from build123d import *

# Parameters (mm, degrees)
BOSS_EXTRUDE1_DEPTH = 88
SKETCH5_W           = 120.314234724
SKETCH5_H           = 205.924557391
CUT_EXTRUDE1_DEPTH  = 88
CUT_EXTRUDE2_REACH  = 78.774


with BuildPart() as part:
    # Sketch2 → Boss-Extrude1 (new body)
    with BuildSketch(Plane.XY):
        Polygon((21.738330866, 28.073521819), (21.738330866, -43.926478181), (-19.131432817, -43.926478181), (-19.989175059, -37.823325008), (7.738330866, -33.926478181), (0.362156515, 18.557729462), (-6.569719966, 17.583517755), (-8.043993893, 28.073521819), align=None)
    extrude(amount=-BOSS_EXTRUDE1_DEPTH)

    # Sketch5 → Cut-Extrude1 (cut)
    with BuildSketch(Plane(origin=(19.710307893, 24.555901932, -20.242027268), x_dir=(-0.850144649, 0.406300724, -0.33492357), z_dir=(-0.526549216, -0.655996394, 0.540753784))):
        with Locations((18.13624664, 41.178747918)):
            Rectangle(SKETCH5_W, SKETCH5_H)
    extrude(amount=-CUT_EXTRUDE1_DEPTH, mode=Mode.SUBTRACT)

    # Cut-Extrude2: up to this face of the body (flat: up to its plane)
    cut_extrude2_end = Plane(part.part.faces().sort_by_distance((4.446485826, -10.503783654, -37.636714234))[0])
    # Sketch6 → Cut-Extrude2 (cut, up to the picked face)
    with BuildSketch(Plane(origin=(19.710307893, 24.555901932, -20.242027268), x_dir=(0.850144649, -0.406300724, 0.33492357), z_dir=(0.526549216, 0.655996394, -0.540753784)), mode=Mode.PRIVATE) as cut_extrude2_sk1:
        with BuildLine():
            Line((-1.614496573, 26.946007892), (-1.614496573, 48.946007892))
            ThreePointArc((-1.614496573, 48.946007892), (-5.614496573, 52.946007892), (-9.614496573, 48.946007892))
            Line((-9.614496573, 48.946007892), (-9.614496573, 26.946007892))
            ThreePointArc((-9.614496573, 26.946007892), (-5.614496573, 22.946007892), (-1.614496573, 26.946007892))
        make_face()
    cut_extrude2_tool1 = split(extrude(cut_extrude2_sk1.sketch, amount=-CUT_EXTRUDE2_REACH, mode=Mode.PRIVATE), bisect_by=cut_extrude2_end, keep=Keep.BOTH, mode=Mode.PRIVATE)
    add(cut_extrude2_tool1.solids().sort_by_distance((14.937174, 2.700657, -51.4027))[0], mode=Mode.SUBTRACT)


solid = part.part
Here's how the part is built. I have some questions about the finished solid (model axes, mm). A direction names the side the tool comes from. Round coordinates to 2 decimals unless told otherwise and drop trailing zeros. Loops run counter-clockwise (first coordinate to the right, second up) from the corner with the lowest first, then second, coordinate; pieces in that order, holes last. Notation, with made-up numbers: M 52,40.5 L 75,40.5 A20 ccw 75,76.5 Z; hole C 37,31 d1. An arc over 180 degrees is marked long. Write each question's results on one line, items separated by ' | '. Start each with the question number.
(1) I want a section at A-A (z = -24). Please give me the cut outline in (x, y).
(2) Thinking about a two-plate mould opening in Z: for faces 1 (the flat face through (3, 28.074, -16)), 2 (the flat face through (10, -7, 0)), 3 (the cylindrical face through (10.644, 4.875, -34.03)), 4 (the flat face through (10.365, 2.582, -55.999)), which applies, pulls with the +Z half, pulls with the -Z half, needs draft (parallel to the pull), parting line crosses it, or undercut?
(3) I want a section at B-B (y = -30). Please give me the cut outline in (x, z).
(4) On a 3-axis mill with a long thin cutter (end or side, diameter ignored), from which of +Z, -Z, +X, -X, +Y, -Y can I reach the whole of each face in a straight line? I mean faces 5 (the flat face through (-3.055, 18.077, -26.765)), 6 (the flat face through (-7.297, 22.755, -26.765)), 7 (the flat face through (11.414, -7.452, -42.834)), 8 (the flat face through (21.738, -15, -34)). Say none if no direction works.
(5) I want a section at C-C (x = -14.5). Please give me the cut outline in (y, z), then the cut area to 3 significant figures.
(6) If I drill on probe 1 along Y at (x, z) = (8, -43.5); probe 2 along X at (y, z) = (1, -27); probe 3 along X at (y, z) = (1.5, -37.5), over which ranges is the centre line in solid material (lowest first)? Write a range as from..to.
(7) I want a section at D-D (z = -71). Please give me the cut outline in (x, y).
(8) Will these pins go through, and if not, where does the flat tip stop? P1, Ø10, axis at y = -26, z = -14, coming from the -X side; P2, Ø6, axis at x = -13, z = -42.5, coming from the +Y side; P3, Ø5, axis at y = -24.5, z = -25.5, coming from the -X side.
Solved:
1) outline: M -19.99,-37.82 L -19.13,-43.93 L 21.74,-43.93 L 21.74,19.83 L 11.47,28.07 L -8.04,28.07 L -6.57,17.58 L 0.36,18.56 L 7.74,-33.93 Z
2) face 1: needs draft | face 2: pulls with the +Z half | face 3: undercut | face 4: pulls with the -Z half
3) outline: M 7.19,-88 L 18.09,-88 L 21.74,-84.45 L 21.74,0 L 7.19,0 Z
4) face 5: +Z, -Z | face 6: +Z, -Z, -X | face 7: none | face 8: +Z, -Z, +X, +Y, -Y
5) outline: M -43.93,-88 L -37.05,-88 L -37.05,0 L -43.93,0 Z | area: 605 mm²
6) probe 1: y = -43.93..-15.15, 4.54..14.78 | probe 2: x = 2.83..21.74 | probe 3: x = 2.76..4.18, 13.59..21.74
7) outline: M -19.99,-37.82 L -19.13,-43.93 L 21.74,-43.93 L 21.74,-18.91 L 3.58,-4.34 L 7.74,-33.93 Z
8) P1: stops at x = 5.92 | P2: stops at y = -36.42 | P3: stops at x = 6.06
